Source: CAD feature listing. Evaluate the final solid. Frame: model axes, mm. Face numbers are marked on the shaded views. A direction names the side the tool comes from. Give positions to 0.01 mm unless a question says otherwise; leave off trailing zeros. Loops run counter-clockwise (first coordinate to the right, second up) from the corner with the lowest first, then second, coordinate; pieces in that order, holes last. Notation, with made-up numbers: M -13.75,16.5 L 16.25,16.5 A29 cw 16.25,40.5 Z; hole C -36.75,31 d1. An arc over 180 degrees is marked long. Answer in a Markdown table with one row per item.
```python
from build123d import *

# Parameters (mm, degrees)
SKETCH1_R           = 1.5
BOSS_EXTRUDE1_DEPTH = 10
SKETCH3_R           = 1.75
CUT_EXTRUDE1_DEPTH  = 6


with BuildPart() as part:
    # Sketch1 → Boss-Extrude1 (new body)
    with BuildSketch(Plane.XY):
        with BuildLine():
            Line((-10, -2.5), (-18, -2.5))
            Line((-18, -2.5), (-20, -7.5))
            Line((-20, -7.5), (20, -7.5))
            Line((20, -7.5), (18, -2.5))
            Line((18, -2.5), (10, -2.5))
            ThreePointArc((10, -2.5), (8.232233047, -1.767766953), (7.5, 0))
            ThreePointArc((7.5, 0), (0, 7.5), (-7.5, 0))
            ThreePointArc((-7.5, 0), (-8.232233047, -1.767766953), (-10, -2.5))
        make_face()
        Circle(SKETCH1_R, mode=Mode.SUBTRACT)
    extrude(amount=BOSS_EXTRUDE1_DEPTH)

    # Sketch2 → Cut-Revolve1 (revolve, cut)
    with BuildSketch(Plane(origin=(0, 0, 0), x_dir=(1, 0, 0), z_dir=(0, 1, 0))):
        Polygon((0, 0), (0, -5), (4, 0), align=None)
        Polygon((2.7, -5), (1.5, -5), (1.5, -3.125), (0, -5), (0, -10), (2.7, -10), align=None)
    revolve(axis=Axis((0, 0, 0), (0, 0, 1)), mode=Mode.SUBTRACT)

    # Sketch3 → Cut-Extrude1 (cut, through all)
    with BuildSketch(Plane(origin=(0, -2.5, 0), x_dir=(1, 0, 0), z_dir=(0, 1, 0))):
        with Locations((-14, -5)):
            Circle(SKETCH3_R)
        with Locations((14, -5)):
            Circle(SKETCH3_R)
    extrude(amount=-CUT_EXTRUDE1_DEPTH, mode=Mode.SUBTRACT)


solid = part.part
```
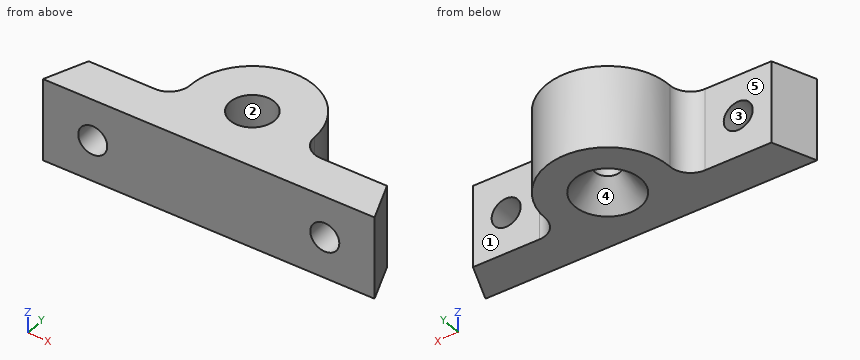
1) Section A-A, the plane x = 14. Return loops of the section in (y, z), then the cut area to 3 significant figures.
Reply:
| item | result |
|---|---|
| outline | M -7.5,0 L -2.5,0 L -2.5,3.25 L -7.5,3.25 Z; M -7.5,6.75 L -2.5,6.75 L -2.5,10 L -7.5,10 Z |
| area | 32.5 mm² |
2) Pull-direction query (Y, two-part tool) for the marked faces 1, 2 and 3; classes: released by +Y, released by -Y, zero draft, split by the parting line, or undercut.
Reply:
| item | result |
|---|---|
| face 1 | released by +Y |
| face 2 | undercut |
| face 3 | zero draft |
3) Section B-B, the plane z = 1. Return loops of the section in (x, y), then the cut area to 3 significant figures.
Reply:
| item | result |
|---|---|
| outline | M -20,-7.5 L 20,-7.5 L 18,-2.5 L 10,-2.5 A2.5 cw 7.5,0 A7.5 ccw -7.5,0 A2.5 cw -10,-2.5 L -18,-2.5 Z; hole C 0,0 d6.4 |
| area | 286 mm² |
4) Section C-C, the plane y = -6. Return loops of the section in (x, z).
Reply:
| item | result |
|---|---|
| outline | M -19.4,0 L 19.4,0 L 19.4,10 L -19.4,10 Z; hole C -14,5 d3.5; hole C 14,5 d3.5 |
5) Pin query (flat end, axial travel): pin 1 Ø4 at (x, z) = (4, 2.5) entering from +Y; pin 2 Ø2.5 at (x, y) = (0, 0) entering from +Z; pin 3 Ø3 at (x, z) = (14, 4.5) entering from +Y; pin 4 Ø5 at (y, z) = (-1, 7) entering from +X. Return the tip coordinate at first contact, or that it passes through.
Reply:
| item | result |
|---|---|
| pin 1 | stops at y = 7.23 |
| pin 2 | passes through |
| pin 3 | stops at y = -2.5 |
| pin 4 | stops at x = 18.4 |
6) Set-up query: the marked faces 4 and 5. Return all of +Z, -Z, +X, -X, +Y, -Y with unobstructed straight access to the full face (end or side cutting, diameter ignored); none if empty.
Reply:
| item | result |
|---|---|
| face 4 | -Z |
| face 5 | +Z, -Z, -X, +Y |
7) Material intervals for L1, parallel to X at y = -3.8, z = 5; L2, parallel to Y at x = 0, z = 3.8; L3, parallel to Z at x = 14, y = -3.5, sorted ascending.
Reply:
| item | result |
|---|---|
| L1 | x = -18.52 to -15.75, -12.25 to 12.25, 15.75 to 18.52 |
| L2 | y = -7.5 to -1.5, 1.5 to 7.5 |
| L3 | z = 0 to 3.25, 6.75 to 10 |
8) Section D-D, the plane z = 3.75. Return loops of the section in (x, y).
Reply:
| item | result |
|---|---|
| outline | M -20,-7.5 L -15.22,-7.5 L -15.22,-2.5 L -18,-2.5 Z; M -12.78,-7.5 L 12.78,-7.5 L 12.78,-2.5 L 10,-2.5 A2.5 cw 7.5,0 A7.5 ccw -7.5,0 A2.5 cw -10,-2.5 L -12.78,-2.5 Z; M 15.22,-7.5 L 20,-7.5 L 18,-2.5 L 15.22,-2.5 Z; hole C 0,0 d3 |
